Read the model definition and answer for the solid it produces. Units are mm, in the model's axes. A direction names the side the tool comes from. Coordinates: 2 decimals unless noted, no trailing zeros. Write each loop counter-clockwise with the first axis right and the second up, starting at its lowest first coordinate (ties: lowest second). Pieces come first, ordered by that corner, then holes. Notation, with made-up numbers: (-11, 9) -> (42, 9) arc R16 ccw to (42, 35) -> close; hole circle Ø11 at (5.5, 69). An arc over 180 degrees is marked (long way). Return JSON: item names as keys, results as strings.
Autodesk Inventor part; units mm, degrees
ref_plane "Work Plane2" through (-20, -20, -70) normal (0, 0, -1) x (0, 1, 0)
ref_plane "Work Plane3" through (-25, -81.8654, -89) normal (0, 0, -1) x (0, 1, 0)
ref_plane "YZ Plane" through (0, 0, 0) normal (1, 0, 0) x (0, 1, 0)
ref_plane "Work Plane1" through (0, 0, 0) normal (0, 0, 1) x (1, 0, 0)
sketch "Sketch1" plane through (0, 0, 0) normal (0, 0, 1) x (1, 0, 0)
  circle A0 centre (0, -19) radius 4.7
  circle A1 centre (19, 0) radius 4.7
  circle A2 centre (0, 19) radius 4.7
  circle A3 centre (-19, 0) radius 4.7
  circle A4 centre (0, 0) radius 13.5
  circle A5 centre (-13.435, 13.435) radius 4.7
  circle A6 centre (13.435, 13.435) radius 4.7
  circle A7 centre (13.435, -13.435) radius 4.7
  circle A8 centre (-13.435, -13.435) radius 4.7
  circle A9 centre (0, 0) radius 13.15
  point P0 (0, 0)
  dimension "d0" = 0.35
  dimension "d16" = 9.4
  dimension "d17" = 27
  dimension "d18" = 14.542
  dimension "d19" = 14.542
  dimension "d20" = 26.8701
  dimension "d21" = 19
  dimension "d22" = 26.8701
  dimension "d23" = 35.1074
  dimension "d24" = 38
  dimension "d25" = 26.8701
  dimension "d26" = 14.542
  dimension "d27" = 19
  dimension "d28" = 35.1074
  dimension "d29" = 26.8701
  dimension "d30" = 35.1074
  dimension "d31" = 38
  dimension "d32" = 26.8701
ref_plane "Work Plane2" through (-20, -20, -70) normal (0, 0, -1) x (0, 1, 0)
ref_plane "Work Plane3" through (-25, -81.8654, -89) normal (0, 0, -1) x (0, 1, 0)
extrude "Extrusion1" add sketch "Sketch1" against normal blind 90 contours A9
move faces "Move1" translate (0, 0, 3) faces at (-4.0086, 0.988, 0)
sketch "Sketch5" plane through (0, 0, 3) normal (0, 0, 1) x (1, 0, 0)
  circle A0 centre (0, 0) radius 10
  point P0 (0, 0)
  dimension "d11" = 20
extrude "Extrusion4" add sketch "Sketch5" along normal blind 4
sketch "Sketch6" plane through (0, 0, 7) normal (0, 0, 1) x (1, 0, 0)
  circle A0 centre (0, 0) radius 13.15
  point P0 (0, 0)
extrude "Extrusion5" add sketch "Sketch6" along normal blind 4
sketch "Sketch7" plane through (0, 0, -90) normal (0, 0, -1) x (-1, 0, 0)
  circle A0 centre (0, 0) radius 13.15
  circle A1 centre (0, 0) radius 10
  point P0 (0, 0)
  dimension "d35" = 20
extrude "Extrusion6" add sketch "Sketch7" along normal blind 4 contours A1
sketch "Sketch8" plane through (0, 0, -94) normal (0, 0, -1) x (-1, 0, 0)
  circle A0 centre (0, 0) radius 13.15
  point P0 (0, 0)
extrude "Extrusion7" add sketch "Sketch8" along normal blind 4
properties part number "axle-upper_3DPrint"
1. The part is cut by section A-A (y = 0). Determine the outline of the cut face in (x, z), then the cut area to 3 significant figures.
Taken from the geometry:
{"outline": "(-13.15, -98) -> (13.15, -98) -> (13.15, -94) -> (10, -94) -> (10, -90) -> (13.15, -90) -> (13.15, 3) -> (10, 3) -> (10, 7) -> (13.15, 7) -> (13.15, 11) -> (-13.15, 11) -> (-13.15, 7) -> (-10, 7) -> (-10, 3) -> (-13.15, 3) -> (-13.15, -90) -> (-10, -90) -> (-10, -94) -> (-13.15, -94) -> close", "area": "2,820 mm2"}
2. Consider L1, parallel to Z at x = -8.5, y = 9.5; L2, parallel to Y at x = 3.75, z = -21; L3, parallel to X at y = 1.5, z = -77. Determine where each line is inside the solid, lowest interval first.
Taken from the geometry:
{"L1": "z = -98 to -94, -90 to 3, 7 to 11", "L2": "y = -12.6 to 12.6", "L3": "x = -13.06 to 13.06"}
3. A tool of negligible diameter and unlimited length cuts with its end or side. For faces 1 (the face through (-2, 10, 7)), 2 (the face through (13.137, -0.578, -95.972)), from which of +Z, -Z, +X, -X, +Y, -Y can it reach the whole face along a straight path? Write none if from no direction.
Taken from the geometry:
{"face 1": "none", "face 2": "+Z, -Z"}
4. The part is cut by section C-C (z = -71). Determine the outline of the cut face in (x, y), then the cut area to 3 significant figures.
Taken from the geometry:
{"outline": "circle Ø26.3 at (0, 0)", "area": "543 mm2"}
5. Flat-ended cylindrical pins translate along their axes: pin 1 Ø5 at (y, z) = (-2.5, -46) entering from -X; pin 2 Ø5 at (y, z) = (5, -41) entering from -X; pin 3 Ø6 at (x, z) = (9, -61.5) entering from +Y; pin 4 Ø10 at (x, z) = (9.5, -75.5) entering from +Y. Find the tip coordinate at first contact, or state that the pin passes through.
Taken from the geometry:
{"pin 1": "stops at x = -13.15", "pin 2": "stops at x = -12.91", "pin 3": "stops at y = 11.7", "pin 4": "stops at y = 12.36"}
6. For a pull along Z with two mould halves and no side action, classify faces 3 (the face through (-13.137, 0.578, -42.849)), 4 (the face through (-2, 10, -90)), 5 (the face through (0, 0, 11)) as +Z half, -Z half, draft (parallel to the pull), parting line (faces both ways), or undercut.
Taken from the geometry:
{"face 3": "draft", "face 4": "undercut", "face 5": "+Z half"}
